Part model, mm, in its own coordinate system. A direction names the side the tool comes from. Round coordinates to 2 decimals unless told otherwise and drop trailing zeros. Write each loop counter-clockwise with the first axis right and the second up, starting at its lowest first coordinate (ties: lowest second). Pieces come first, ordered by that corner, then holes. Notation, with made-up numbers: M 89,-9.5 L 147,-9.5 A30 cw 147,27.5 Z; hole C 20,81 d5. An arc over 180 degrees is marked long. Answer as a JSON object with one key per item and string values. Group by question number.
1. Two-plate mould, pull along X, no slides. Class faces 4 (the face through (-5, 11.4, 3.6)), 5 (the face through (-58.905, 0.136, -0.867)), 6 (the face through (27, 0, -10)): +X half, -X half, draft (parallel to the pull), parting line (faces both ways), or undercut.
2. Drop flat-ended pins along their axis: pin 1 (1 mm diameter, centred on x = 18, z = 3, fed in from -Y); pin 2 (5 mm diameter, centred on y = 8.5, z = -10.5, fed in from +X); pin 3 (3 mm diameter, centred on x = 11.5, y = -1, fed in from +Z). Give the stop position or say it passes through.
3. Which spindle directions (+Z, -Z, +X, -X, +Y, -Y) get a long thin tool onto all of the face, cutting with end or side? Do faces 1 (the face through (-2.535, 17.084, -3.794)), 2 (the face through (-35.392, -2.914, 9.252)), 3 (the face through (0, 8, -8)). Say none if no direction does.
4. Band-saw the part on A-A, the plane z = 0. Write the cut outline in (x, y), plus the area to 3 significant figures.
5. Drill centre lines: line 1 (X direction, y = -5.5, z = 0); line 2 (X direction, y = -13, z = 9.5); line 3 (Y direction, x = -49.5, z = 0). Where is each one in solid material? Low to high. Write a range as from..to.
6. Band-saw the part on B-B, the plane y = 0. Write the cut outline in (x, z), plus the area to 3 significant figures.
7. Band-saw the part on D-D, the plane x = -55. Write the cut outline in (y, z), plus the area to 3 significant figures.
8. Band-saw the part on C-C, the plane x = -9. Write the cut outline in (y, z), plus the area to 3 significant figures.
from build123d import *

# Parameters (mm, degrees)
CONG_1_R                     = 2
ESQUISSE2_R                  = 4
ENL_V_MAT_EXTRU_1_DEPTH      = 18.5
ENL_V_MAT_EXTRU_1_DEPTH_BACK = 18.5


with BuildPart() as part:
    # Esquisse1 → Révolution1 (revolve)
    with BuildSketch(Plane.XY, mode=Mode.PRIVATE) as r_volution1_sk:
        Polygon((55, 0), (55, 10), (0, 10), (0, 17.5), (-5, 17.5), (-5, 9.7), (-63, 9.7), (-65, 7.7), (-65, 0), align=None)
    revolve(r_volution1_sk.sketch.rotate(Axis((0, 0, 0), (1, 0, 0)), 90), axis=Axis((0, 0, 0), (1, 0, 0)))  # turned: the seam where the file's is

    # Congé1
    cong_1_edges = [part.edges().sort_by_distance(p)[0] for p in [
        (-5, 0, -9.7),
    ]]
    fillet(cong_1_edges, radius=CONG_1_R)

    # Esquisse2 → Enlèv. mat.-Extru.1 (cut, two sides)
    with BuildSketch(Plane(origin=(0, 0, 0), x_dir=(1, 0, 0), z_dir=(0, 1, 0))) as enl_v_mat_extru_1_sk:
        with Locations(Location((-55, 0, 0), (0, 0, 270))):  # turned: the seam where the file's is
            Circle(ESQUISSE2_R)
    extrude(amount=ENL_V_MAT_EXTRU_1_DEPTH, mode=Mode.SUBTRACT)
    extrude(enl_v_mat_extru_1_sk.sketch, amount=-ENL_V_MAT_EXTRU_1_DEPTH_BACK, mode=Mode.SUBTRACT)


solid = part.part
Worked answers:
{
 "1": {"face 4": "-X half", "face 5": "undercut", "face 6": "draft"},
 "2": {"pin 1": "stops at y = -9.68", "pin 2": "stops at x = 0", "pin 3": "stops at z = 10"},
 "3": {"face 1": "+X, -X", "face 2": "-X", "face 3": "+X"},
 "4": {"outline": "M -65,-7.7 L -63,-9.7 L -59,-9.7 L -59,9.7 L -63,9.7 L -65,7.7 Z; M -51,-9.7 L -7,-9.7 A2 cw -5,-11.7 L -5,-17.5 L 0,-17.5 L 0,-10 L 55,-10 L 55,10 L 0,10 L 0,17.5 L -5,17.5 L -5,11.7 A2 cw -7,9.7 L -51,9.7 Z", "area": "2,280 mm^2"},
 "5": {"line 1": "x = -65..-59, -51..55", "line 2": "x = -5..0", "line 3": "y = -9.7..9.7"},
 "6": {"outline": "M -65,-7.7 L -63,-9.7 L -7,-9.7 A2 cw -5,-11.7 L -5,-17.5 L 0,-17.5 L 0,-10 L 55,-10 L 55,10 L 0,10 L 0,17.5 L -5,17.5 L -5,11.7 A2 cw -7,9.7 L -63,9.7 L -65,7.7 Z; hole C -55,0 d8", "area": "2,390 mm^2"},
 "7": {"outline": "M -8.84,-4 A9.7 ccw 8.84,-4 Z; M -8.84,4 L 8.84,4 A9.7 ccw Z", "area": "145 mm^2"},
 "8": {"outline": "C 0,0 d19.4", "area": "296 mm^2"}
}
